The model under review builds one solid part; all positions refer to its coordinate system, in mm. A direction names the side the tool comes from. Coordinates: 2 decimals unless noted, no trailing zeros. Order: outer loops, then holes, each group sorted by start corner. A loop starts at its lowest first (then second) coordinate and runs counter-clockwise, first axis right, second up. Notation, with made-up numbers: M -12.5,-30.75 L 42.5,-30.75 A19 ccw 42.5,-20.75 Z; hole C -2,20.5 d4. An arc over 180 degrees is marked long. Answer in a Markdown table with one row per item.
from build123d import *

# Parameters (mm, degrees)
F0_R     = 9.525
F1_DEPTH = 25.4
F2_R     = 25.4
F3_DEPTH = 25.4
F4_R     = 12.7
F5_DEPTH = 25.4


with BuildPart() as f1:
    # F0 (on Top) → F1 (new body)
    with BuildSketch(Plane.XY):
        with BuildLine():
            ThreePointArc((-12.7, 0), (0, -12.7), (12.7, 0))
            ThreePointArc((12.7, 0), (0, 12.7), (-12.7, 0))
        make_face()
        Circle(F0_R, mode=Mode.SUBTRACT)
        with BuildLine():
            ThreePointArc((-12.7, 0), (0, 12.7), (12.7, 0))
            Line((12.7, 0), (12.7, 177.8))
            Line((12.7, 177.8), (-12.7, 177.8))
            Line((-12.7, 177.8), (-12.7, 0))
        make_face()
    extrude(amount=F1_DEPTH)

    # F2 (on face) → F3 (join)
    with BuildSketch(Plane.XY.offset(25.4)):
        with Locations((0, 177.8)):
            Circle(F2_R)
    extrude(amount=-F3_DEPTH)

    # F4 (on face) → F5 (cut)
    with BuildSketch(Plane.XY.offset(25.4)):
        with Locations((0, 177.8)):
            Circle(F4_R)
    extrude(amount=-F5_DEPTH, mode=Mode.SUBTRACT)


solid = f1.part
(1) Insertion check: P1, Ø5, axis at y = 9.5, z = 6.5, coming from the +X side; P2, Ø5, axis at y = 169.5, z = 14.5, coming from the +X side; P3, Ø6, axis at y = 140.5, z = 9.5, coming from the -X side. Each pin has a flat end and moves straight along its axis. Give the tip position at first contact, or say it passes through.
Report:
| item | result |
|---|---|
| P1 | x = 12.7 |
| P2 | x = 24.73 |
| P3 | x = -12.7 |
(2) The part is to be moulded in two halves that separate along X. For faces 1 (the cylindrical face through (6.827, 188.509, 12.878)), 2 (the flat face through (0, 121, 25.4)), 3 (the flat face through (-12.7, 79, 13)), 4 (the cylindrical face through (-7.559, -5.796, 12.522)), say which applies: +X half, -X half, draft (parallel to the pull), parting line (faces both ways), or undercut.
Report:
| item | result |
|---|---|
| face 1 | undercut |
| face 2 | draft |
| face 3 | -X half |
| face 4 | undercut |
(3) Take a section at C-C (z = 21.25). Write out the cut boundary in (x, y) (3 decimals), then the cut area to 3 significant figures.
Report:
| item | result |
|---|---|
| outline | M -12.7,0 A12.7 ccw 12.7,0 L 12.7,155.803 A25.4 ccw long -12.7,155.803 Z; hole C 0,177.8 d25.4; hole C 0,0 d19.05 |
| area | 5,390 mm^2 |
(4) Take a section at B-B (x = 0). Write out the cut boundary in (y, z) (3 decimals).
Report:
| item | result |
|---|---|
| outline | M -12.7,0 L -9.525,0 L -9.525,25.4 L -12.7,25.4 Z; M 9.525,0 L 165.1,0 L 165.1,25.4 L 9.525,25.4 Z; M 190.5,0 L 203.2,0 L 203.2,25.4 L 190.5,25.4 Z |
(5) Machinability: for faces 5 (the flat face through (12.7, 77, 13)), 6 (the flat face through (0, 121, 0)), which of the approach directions +Z, -Z, +X, -X, +Y, -Y give a long, thin tool a straight path to every point of the face, cutting with its end or side? Answer none if there is none.
Report:
| item | result |
|---|---|
| face 5 | +Z, -Z, +X, -Y |
| face 6 | -Z, +X, -X, +Y, -Y |
(6) Take a section at D-D (y = 109). Write out the cut boundary in (x, z), then the cut area to 3 significant figures.
Report:
| item | result |
|---|---|
| outline | M -12.7,0 L 12.7,0 L 12.7,25.4 L -12.7,25.4 Z |
| area | 645 mm^2 |
(7) To check wall thickness, follow line 1 (Y direction, x = 0, z = 10.5) (3 decimals); line 2 (Y direction, x = -11.5, z = 10); line 3 (Y direction, x = 2, z = 19.5). State the ranges of each line that lie inside material, in increasing order. Write a range as [from, to].
Report:
| item | result |
|---|---|
| line 1 | [-12.7, -9.525], [9.525, 165.1], [190.5, 203.2] |
| line 2 | [-5.39, 172.41], [183.19, 200.45] |
| line 3 | [-12.54, -9.31], [9.31, 165.26], [190.34, 203.12] |
(8) Take a section at A-A (y = 177.8). Write out the cut boundary in (x, z), then the cut area to 3 significant figures.
Report:
| item | result |
|---|---|
| outline | M -25.4,0 L -12.7,0 L -12.7,25.4 L -25.4,25.4 Z; M 12.7,0 L 25.4,0 L 25.4,25.4 L 12.7,25.4 Z |
| area | 645 mm^2 |
